Verification items for the finished model (mm, model axes). Coordinates: 2 decimals unless noted, no trailing zeros. Order: outer loops, then holes, each group sorted by start corner. A loop starts at its lowest first (then second) coordinate and runs counter-clockwise, first axis right, second up.
Q1. Depth check by flat-ended pin: P1, Ø2.5, axis at x = 0, z = 0, coming from the -Y side. Enter the tip coordinate at first touch or a pass-through.
Q2. Cross-section at A-A, the plane y = 3.4. Record the boundary of the cut face in (x, z).
Q3. Cross-section at C-C, the plane z = -0.3. Record the boundary of the cut face in (x, y), and give its area (3 significant figures).
Q4. Draft check along X on faces 1 (the flat face through (0, 2, 2.3)), 2 (the cylindrical face through (0.45, 1.97, -1.43)), 3 (the flat face through (-2.001, 1.972, 1.134)), 4 (the flat face through (1.98, 1.97, 1.17)). Enter one of: pulls with the +X half, pulls with the -X half, needs draft (parallel to the pull), parting line crosses it, or undercut.
Q5. Cross-section at B-B, the plane x = 0. Record the boundary of the cut face in (y, z), and give its area (3 significant figures).
Q6. Cross-section at D-D, the plane x = 2.2. Record the boundary of the cut face in (y, z), and give its area (3 significant figures).
Q7. Thickness scan on line 1 (X direction, y = 1.4, z = -1.2); line 2 (Z direction, x = 0.35, y = 0.3); line 3 (X direction, y = 1.1, z = -1.15). Record the ranges inside material, lowest first.
from build123d import *

# Parameters (mm, degrees)
EXTRUDE_1_DEPTH     = 4
SKETCH_4_R          = 1.5
CUT_EXTRUDE_1_DEPTH = 4


with BuildPart() as part:
    # 草图1 → 凸台-拉伸1 (new body)
    with BuildSketch(Plane(origin=(0, 0, 0), x_dir=(1, 0, 0), z_dir=(0, 1, 0))):
        Polygon((-1.327905619, 2.3), (-2.655811238, 0), (-1.327905619, -2.3), (1.327905619, -2.3), (2.655811238, 0), (1.327905619, 2.3), align=None)
    extrude(amount=EXTRUDE_1_DEPTH)

    # 草图4 → 切除-拉伸1 (cut)
    with BuildSketch(Plane.XZ):
        with Locations(Location((0, 0, 0), (0, 0, 270))):
            Circle(SKETCH_4_R)
    extrude(amount=-CUT_EXTRUDE_1_DEPTH, mode=Mode.SUBTRACT)


solid = part.part
Check values:
1. P1: passes through
2. outline: (-2.66, 0) - (-1.33, -2.3) - (1.33, -2.3) - (2.66, 0) - (1.33, 2.3) - (-1.33, 2.3) - close; hole circle Ø3 at (0, 0)
3. outline: (-2.48, 0) - (-1.47, 0) - (-1.47, 4) - (-2.48, 4) - close; (1.47, 0) - (2.48, 0) - (2.48, 4) - (1.47, 4) - close
3. area: 8.10 mm2
4. face 1: needs draft
4. face 2: undercut
4. face 3: pulls with the -X half
4. face 4: pulls with the +X half
5. outline: (0, -2.3) - (4, -2.3) - (4, -1.5) - (0, -1.5) - close; (0, 1.5) - (4, 1.5) - (4, 2.3) - (0, 2.3) - close
5. area: 6.40 mm2
6. outline: (0, -0.79) - (4, -0.79) - (4, 0.79) - (0, 0.79) - close
6. area: 6.32 mm2
7. line 1: x = -1.96 to -0.9, 0.9 to 1.96
7. line 2: z = -2.3 to -1.46, 1.46 to 2.3
7. line 3: x = -1.99 to -0.96, 0.96 to 1.99
